```python
from build123d import *

# Parameters (mm, degrees)
F0_R        = 5.0651423349
F1_DEPTH    = 50
F2_SIZE2    = 8
F2_SIZE     = 5
F4_T1_DEPTH = 460.97003859


# Not quite as in the source:
# - a fillet or chamfer that OpenCascade refuses, or shapes differently, is made with other operations: its cross-section is extruded or revolved along the edge and cut away or added


with BuildPart() as f1:
    # F0 (on Top) → F1 (new body)
    with BuildSketch(Plane.XY):
        Polygon((-70.2088537009, 12.9954309589), (-70.2088537009, 39.781139965), (-46.9945719463, 39.781139965), (-46.9945719463, 49.781139965), (-96.9945719463, 49.781139965), (-96.9945719463, -5.9331371699), (-46.9945719463, -5.9331371699), (-46.9945719463, 12.9954309589), align=None)
        with Locations((-82.137003541, 20.1600026339)):
            Circle(F0_R, mode=Mode.SUBTRACT)
    extrude(amount=F1_DEPTH)

    # F2
    f2_edges = [f1.edges().sort_by_distance(p)[0] for p in [
        (-96.994572, 21.924001, 50),
    ]]
    f2_side = f1.faces().sort_by_distance((-96.994572, 21.924001, 25))[0]
    chamfer(f2_edges, length=F2_SIZE, length2=F2_SIZE2, reference=f2_side)

    # F3: fillet of radius 15 on 1 edges, made by hand

    # F3_s1 → F3_t2 (revolve, cut)
    with BuildSketch(Plane.XZ.offset(-20.1600026339)):
        with BuildLine():
            ThreePointArc((-62.0718612061, 0), (-72.6784629239, 4.3933982822), (-77.0718612061, 15))
            Line((-77.0718612061, 15), (-77.0718612061, 0))
            Line((-77.0718612061, 0), (-62.0718612061, 0))
        make_face()
    revolve(axis=Axis((-82.137003541, 20.1600026339, 0), (0, 0, 1)), mode=Mode.SUBTRACT)

    # F4: chamfer of 5 x 80 on 1 edges, made by hand

    # F4_s2 → F4_t1 (cut)
    with BuildSketch(Plane.XY.offset(-207.985019295)):
        Polygon((-16.9945719463, 49.781139965), (-96.9945719463, 44.781139965), (-96.9945719463, 49.781139965), align=None)
    extrude(amount=F4_T1_DEPTH, mode=Mode.SUBTRACT)


solid = f1.part
```
The listing builds one solid part. Answer for the finished solid, in the listing's coordinates (mm). A direction names the side the tool comes from. Round coordinates to 2 decimals unless told otherwise and drop trailing zeros. Loops run counter-clockwise (first coordinate to the right, second up) from the corner with the lowest first, then second, coordinate; pieces in that order, holes last. Notation, with made-up numbers: (-32.5, -6.75) - (-23.5, -6.75) arc R30 ccw to (-23.5, 25.25) - close; hole circle Ø2 at (80.5, 14). An arc over 180 degrees is marked (long way). Return JSON: item names as keys, results as strings. Group by question number.
1. The part is cut by section B-B on x = -53.5. Determine the outline of the cut face in (y, z), then the cut area to 3 significant figures.
2. The part is cut by section D-D on z = 4.5. Determine the outline of the cut face in (x, y), then the cut area to 3 significant figures.
3. The part is cut by section A-A on z = 43. Determine the outline of the cut face in (x, y).
4. The part is cut by section C-C on x = -61. Determine the outline of the cut face in (y, z), then the cut area to 3 significant figures.
5. The mould has two halves that part along X. Classify faces 3 (the cylindrical face through (-77.46, 18.22, 32.25)), 4 (the flat face through (-46.995, 3, 25)), 5 (the flat face through (-96.995, 20, 22)), 6 (the flat face through (-72, -5.933, 25)): pulls with the +X half, pulls with the -X half, needs draft (parallel to the pull), parting line crosses it, or undercut.
6. Consider probe 1 along Y at (x, z) = (-62, 24); probe 2 along X at (y, z) = (21, 17.5); probe 3 along Y at (x, z) = (-84, 9). Determine where each line is inside the solid, lowest interval first.
7. Each of these flat-tipped pins is pushed along its axis until it touches: P1, Ø8, axis at x = -59.5, z = 23.5, coming from the +Y side; P2, Ø7, axis at x = -62.5, z = 18, coming from the +Y side; P3, Ø4, axis at y = 36, z = 15.5, coming from the +X side. Where does it stop, or does it pass through?
8. Which of the six approach directions +Z, -Z, +X, -X, +Y, -Y give full straight-line access (tool end or side, diameter ignored) to faces 1 (the flat face through (-58, 12.995, 25)), 2 (the flat face through (-72, 42, 0))?
Resolved:
{
 "1": {"outline": "(-5.93, 0) - (13, 0) - (13, 50) - (-5.93, 50) - close; (39.78, 0) - (47.5, 0) - (47.5, 50) - (39.78, 50) - close", "area": "1,330 mm²"},
 "2": {"outline": "(-96.99, -5.93) - (-46.99, -5.93) - (-46.99, 13) - (-70.21, 13) - (-70.21, 39.78) - (-46.99, 39.78) - (-46.99, 47.91) - (-96.99, 44.78) - close; hole circle Ø18.71 at (-82.14, 20.16)", "area": "1,720 mm²"},
 "3": {"outline": "(-96.99, -5.93) - (-46.99, -5.93) - (-46.99, 13) - (-70.21, 13) - (-70.21, 39.78) - (-46.99, 39.78) - (-46.99, 47.91) - (-96.99, 44.78) - close; hole circle Ø10.13 at (-82.14, 20.16)"},
 "4": {"outline": "(-5.93, 0) - (13, 0) - (13, 50) - (-5.93, 50) - close; (39.78, 0) - (47.03, 0) - (47.03, 50) - (39.78, 50) - close", "area": "1,310 mm²"},
 "5": {"face 3": "undercut", "face 4": "pulls with the +X half", "face 5": "pulls with the -X half", "face 6": "needs draft"},
 "6": {"probe 1": "y = -5.93 to 13, 39.78 to 46.97", "probe 2": "x = -96.99 to -87.13, -77.14 to -70.21", "probe 3": "y = -5.93 to 14.12, 26.2 to 45.59"},
 "7": {"P1": "stops at y = 47.37", "P2": "stops at y = 47.16", "P3": "stops at x = -70.21"},
 "8": {"face 1": "+Z, -Z, +X", "face 2": "-Z, +X, -X, +Y, -Y"}
}
